```python
from build123d import *

# Parameters (mm, degrees)
ESQUISSE1_R             = 27
ESQUISSE1_R_2           = 15.1
BOSS_EXTRU_1_DEPTH      = 15
ESQUISSE2_R             = 20
ENL_V_MAT_EXTRU_1_DEPTH = 12
CONG_1_R                = 2.5


with BuildPart() as part:
    # Esquisse1 → Boss.-Extru.1 (new body)
    with BuildSketch(Plane(origin=(0, 0, 0), x_dir=(1, 0, 0), z_dir=(0, 1, 0))):
        with Locations(Location((0, 0, 0), (0, 0, 270))):  # turned: the seam where the file's is
            Circle(ESQUISSE1_R)
        with Locations(Location((0, 0, 0), (0, 0, 270))):  # turned: the seam where the file's is
            Circle(ESQUISSE1_R_2, mode=Mode.SUBTRACT)
    extrude(amount=BOSS_EXTRU_1_DEPTH)

    # Esquisse2 → Enlèv. mat.-Extru.1 (cut)
    with BuildSketch(Plane(origin=(0, 15, 0), x_dir=(-1, 0, 0), z_dir=(0, 1, 0))):
        with Locations(Location((0, 0, 0), (0, 0, 90))):  # turned: the seam where the file's is
            Circle(ESQUISSE2_R)
    extrude(amount=-ENL_V_MAT_EXTRU_1_DEPTH, mode=Mode.SUBTRACT)

    # Congé1
    cong_1_edges = [part.edges().sort_by_distance(p)[0] for p in [
        (0, 15, -20),
        (0, 0, -27),
        (0, 15, -27),
        (0, 0, -15.1),
    ]]
    fillet(cong_1_edges, radius=CONG_1_R)


solid = part.part
```
Check sheet for the modelled part. Datum: model origin and axes. Units: mm. A direction names the side the tool comes from. Coordinates: 2 decimals unless noted, no trailing zeros. Order: outer loops, then holes, each group sorted by start corner. A loop starts at its lowest first (then second) coordinate and runs counter-clockwise, first axis right, second up. Notation, with made-up numbers: (-37.5, -5) -> (11.5, -5) arc R6 cw to (11.5, 2) -> close; hole circle Ø7 at (56.5, 80). An arc over 180 degrees is marked (long way). Write item = value, one per line. Start each with the question number.
1) Access from +Z, -Z, +X, -X, +Y, -Y to the whole of each face (thin tool, end or side, straight path). Record for faces 1 (the cylindrical face through (-19.524, 7.816, -4.336)), 2 (the flat face through (-20, 15, 11)).
2) Cross-section at C-C (y = 1). Enter the section's corners in (x, z).
3) Cross-section at B-B (x = 0). Enter the section's corners in (y, z).
4) Cross-section at D-D (y = 8.25). Enter the section's corners in (x, z), then the cut area to 3 significant figures.
5) Mould release check, pull along Z, two halves, no side actions. Record for faces 3 (the cylindrical face through (-26.36, 7.43, -5.85)), 4 (the cylindrical face through (-14.74, 2.75, -3.27)), 5 (the flat face through (6, 0, -17)): +Z half, -Z half, draft (parallel to the pull), parting line (faces both ways), or undercut.
6) Go/stop test with flat-tipped pins: P1, Ø18, axis at x = 0, z = 0, coming from the +Y side; P2, Ø3, axis at y = 4, z = 16.5, coming from the -X side; P3, Ø3, axis at x = -5, y = 9, coming from the -Z side; P4, Ø6, axis at y = 4, z = 18.5, coming from the +X side. Record where each tip stops, or that it passes through.
7) Material ranges on L1, parallel to Z at x = 0.5, y = 7.25; L2, parallel to X at y = 14, z = -5; L3, parallel to Z at x = -8, y = 14, recorded low to high.
8) Cross-section at A-A (z = 0). Enter the section's corners in (x, y).
Ans:
q1.face_1 = +Y
q1.face_2 = +Z, -Z, +X, -X, +Y
q2.outline = circle Ø53 at (0, 0); hole circle Ø31.2 at (0, 0)
q3.outline = (0, -24.5) arc R2.5 ccw to (2.5, -27) -> (12.5, -27) arc R2.5 ccw to (15, -24.5) -> (15, -22.5) arc R2.5 ccw to (12.5, -20) -> (3, -20) -> (3, -15.1) -> (2.5, -15.1) arc R2.5 ccw to (0, -17.6) -> close; (0, 17.6) arc R2.5 ccw to (2.5, 15.1) -> (3, 15.1) -> (3, 20) -> (12.5, 20) arc R2.5 ccw to (15, 22.5) -> (15, 24.5) arc R2.5 ccw to (12.5, 27) -> (2.5, 27) arc R2.5 ccw to (0, 24.5) -> close
q4.outline = circle Ø54 at (0, 0); hole circle Ø40 at (0, 0)
q4.area = 1,030 mm²
q5.face_3 = parting line
q5.face_4 = undercut
q5.face_5 = draft
q6.P1 = through
q6.P2 = -22.45
q6.P3 = -26.77
q6.P4 = 22.11
q7.L1 = -27 to -19.99, 19.99 to 27
q7.L2 = -26.02 to -19.88, 19.88 to 26.02
q7.L3 = -25.26 to -18.87, 18.87 to 25.26
q8.outline = (-27, 2.5) arc R2.5 ccw to (-24.5, 0) -> (-17.6, 0) arc R2.5 ccw to (-15.1, 2.5) -> (-15.1, 3) -> (-20, 3) -> (-20, 12.5) arc R2.5 ccw to (-22.5, 15) -> (-24.5, 15) arc R2.5 ccw to (-27, 12.5) -> close; (15.1, 2.5) arc R2.5 ccw to (17.6, 0) -> (24.5, 0) arc R2.5 ccw to (27, 2.5) -> (27, 12.5) arc R2.5 ccw to (24.5, 15) -> (22.5, 15) arc R2.5 ccw to (20, 12.5) -> (20, 3) -> (15.1, 3) -> close
